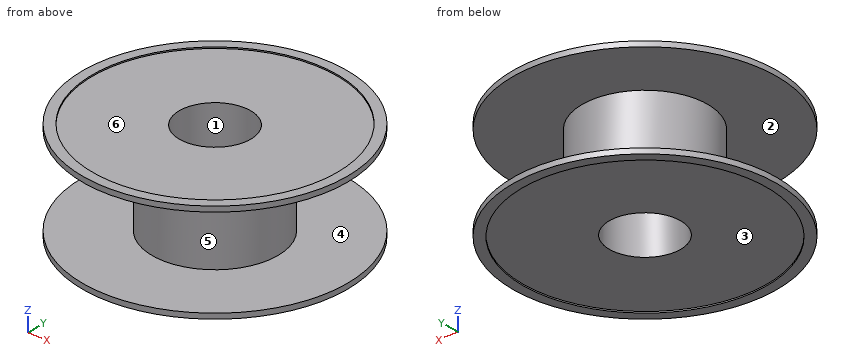
Autodesk Inventor part; units mm, degrees
ref_plane "Work Plane1" through (0, 0, -33.5) normal (0, 0, -1) x (-1, 0, 0)
ref_plane "YZ Plane" through (0, 0, 0) normal (1, 0, 0) x (0, 1, 0)
ref_plane "XZ Plane" through (0, 0, 0) normal (0, 1, 0) x (-1, 0, 0)
sketch "Sketch11" plane through (0, 0, 0) normal (0, 0, 1) x (1, 0, 0)
  circle A0 centre (0, 0) radius 100
  dimension "d39" = 200
extrude "Extrusion10" add sketch "Sketch11" along normal blind 4
sketch "Sketch12" plane through (0, 0, 4) normal (0, 0, 1) x (1, 0, 0)
  circle A0 centre (0, 0) radius 100
  circle A1 centre (0, 0) radius 92.5
  dimension "d42" = 185
extrude "Extrusion11" cut sketch "Sketch12" against normal blind 1 contours A1
ref_plane "Work Plane1" through (0, 0, -33.5) normal (0, 0, -1) x (-1, 0, 0)
mirror "Mirror1" about plane through (0, 0, -33.5) normal (0, 0, -1)
sketch "Sketch14" plane through (0, 0, -67) normal (0, 0, 1) x (1, 0, 0)
  circle A0 centre (0, 0) radius 100
  circle A1 centre (0, 0) radius 47.5
  dimension "d46" = 95
extrude "Extrusion12" add sketch "Sketch14" along normal up to next contours A1
sketch "Sketch15" plane through (0, 0, -70) normal (0, 0, -1) x (-1, 0, 0)
  circle A0 centre (0, 0) radius 92.5
  circle A1 centre (0, 0) radius 27
  dimension "d50" = 54
extrude "Extrusion13" cut sketch "Sketch15" against normal up to surface (73 mm away) contours A1
properties part number "SpoolFilament" material "ABS Plastic"
Read the model definition and answer for the solid it produces. Units are mm, in the model's axes. Face numbers are marked on the shaded views. A direction names the side the tool comes from. Coordinates: 2 decimals unless noted, no trailing zeros. Write each loop counter-clockwise with the first axis right and the second up, starting at its lowest first coordinate (ties: lowest second). Pieces come first, ordered by that corner, then holes. Notation, with made-up numbers: M 23,-38.5 L 38,-38.5 A26 cw 38,-22.5 Z; hole C 71.25,75.5 d6. An arc over 180 degrees is marked long. Use a Markdown table: item, result.
Q1. The part is cut by section D-D, the plane y = -30.5. Write down the section's boundary in (x, z).
Answer block:
| item | result |
|---|---|
| outline | M -95.24,-71 L -87.33,-71 L -87.33,-70 L 87.33,-70 L 87.33,-71 L 95.24,-71 L 95.24,-67 L 36.41,-67 L 36.41,0 L 95.24,0 L 95.24,4 L 87.33,4 L 87.33,3 L -87.33,3 L -87.33,4 L -95.24,4 L -95.24,0 L -36.41,0 L -36.41,-67 L -95.24,-67 Z |
Q2. Determine the mould class of the marked faces 3, 4, 5 and 6 for opening direction Y: released by +Y, released by -Y, zero draft, split by the parting line, or undercut.
Answer block:
| item | result |
|---|---|
| face 3 | undercut |
| face 4 | zero draft |
| face 5 | split by the parting line |
| face 6 | undercut |
Q3. Straight lines are drawn through the part: L1, parallel to Z at x = -35.5, y = 82; L2, parallel to Y at x = 0, z = -51.5; L3, parallel to Y at x = 0, z = -70.2. For each, find the intervals that lie inside material, in ascending order. Write a range as [from, to].
Answer block:
| item | result |
|---|---|
| L1 | z = [-70, -67], [0, 3] |
| L2 | y = [-47.5, -27], [27, 47.5] |
| L3 | y = [-100, -92.5], [92.5, 100] |
Q4. The part is cut by section A-A, the plane y = 0. Write down the section's boundary in (x, z), then the cut area to 3 significant figures.
Answer block:
| item | result |
|---|---|
| outline | M -100,-71 L -92.5,-71 L -92.5,-70 L -27,-70 L -27,3 L -92.5,3 L -92.5,4 L -100,4 L -100,0 L -47.5,0 L -47.5,-67 L -100,-67 Z; M 27,-70 L 92.5,-70 L 92.5,-71 L 100,-71 L 100,-67 L 47.5,-67 L 47.5,0 L 100,0 L 100,4 L 92.5,4 L 92.5,3 L 27,3 Z |
| area | 3,650 mm2 |
Q5. Each of these flat-tipped pins is pushed along its axis until it touches: pin 1 Ø8 at (x, y) = (13, 33.5) entering from -Z; pin 2 Ø5 at (x, z) = (-14.5, -14) entering from +Y; pin 3 Ø2 at (x, z) = (-13.5, -29.5) entering from +Y. Where does it stop, or does it pass through?
Answer block:
| item | result |
|---|---|
| pin 1 | stops at z = -70 |
| pin 2 | stops at y = 45.96 |
| pin 3 | stops at y = 45.83 |
Q6. Which of the six approach directions +Z, -Z, +X, -X, +Y, -Y give full straight-line access (tool end or side, diameter ignored) to the marked faces 1 and 2?
Answer block:
| item | result |
|---|---|
| face 1 | +Z, -Z |
| face 2 | none |
Q7. The part is cut by section C-C, the plane z = -25. Write down the section's boundary in (x, y), then the cut area to 3 significant figures.
Answer block:
| item | result |
|---|---|
| outline | C 0,0 d95; hole C 0,0 d54 |
| area | 4,800 mm2 |
